Can you work these out from the model? Positions are in its coordinate system, mm. A direction names the side the tool comes from. Coordinates: 2 decimals unless noted, no trailing zeros. Loops run counter-clockwise (first coordinate to the right, second up) from the corner with the lowest first, then second, coordinate; pieces in that order, holes last. Notation, with made-up numbers: M 28.25,43 L 33.25,43 A29 ccw 33.25,73 Z; hole C -19,43 d8. An arc over 180 degrees is marked long. Return JSON: item names as keys, results as strings. Group by question number.
```python
from build123d import *

# Parameters (mm, degrees)
SKETCH1_W           = 119
SKETCH1_H           = 40
BOSS_EXTRUDE1_DEPTH = 4
SKETCH2_W           = 125
SKETCH2_H           = 46
SKETCH2_W_2         = 119
SKETCH2_H_2         = 40
BOSS_EXTRUDE2_DEPTH = 44
SKETCH3_W           = 58.2
SKETCH3_H           = 40
BOSS_EXTRUDE3_DEPTH = 3
SKETCH4_W           = 28
SKETCH4_H           = 40
BOSS_EXTRUDE4_DEPTH = 1.5
SKETCH5_R           = 4
BOSS_EXTRUDE5_DEPTH = 12
SKETCH6_R           = 11.5
SKETCH6_R_2         = 4
CUT_EXTRUDE1_DEPTH  = 3
SKETCH7_R           = 11.5
SKETCH7_R_2         = 9
CUT_EXTRUDE2_DEPTH  = 1


with BuildPart() as part:
    # Sketch1 → Boss-Extrude1 (new body)
    with BuildSketch(Plane(origin=(0, 0, 0), x_dir=(1, 0, 0), z_dir=(0, 1, 0))):
        Rectangle(SKETCH1_W, SKETCH1_H)
    extrude(amount=BOSS_EXTRUDE1_DEPTH)

    # Sketch2 → Boss-Extrude2 (add)
    with BuildSketch(Plane(origin=(0, 0, 0), x_dir=(1, 0, 0), z_dir=(0, 1, 0))):
        Rectangle(SKETCH2_W, SKETCH2_H)
        Rectangle(SKETCH2_W_2, SKETCH2_H_2, mode=Mode.SUBTRACT)
    extrude(amount=BOSS_EXTRUDE2_DEPTH)

    # Sketch3 → Boss-Extrude3 (add)
    with BuildSketch(Plane(origin=(0, 4, 0), x_dir=(1, 0, 0), z_dir=(0, 1, 0))):
        with Locations((30.4, 0)):
            Rectangle(SKETCH3_W, SKETCH3_H)
    extrude(amount=BOSS_EXTRUDE3_DEPTH)

    # Sketch4 → Boss-Extrude4 (add)
    with BuildSketch(Plane(origin=(0, 7, 0), x_dir=(1, 0, 0), z_dir=(0, 1, 0))):
        with Locations((15.3, 0)):
            Rectangle(SKETCH4_W, SKETCH4_H)
    extrude(amount=BOSS_EXTRUDE4_DEPTH)

    # Sketch5 → Boss-Extrude5 (add)
    with BuildSketch(Plane.XZ):
        with Locations((39.5, 0)):
            Circle(SKETCH5_R)
    extrude(amount=BOSS_EXTRUDE5_DEPTH)

    # Sketch6 → Cut-Extrude1 (cut)
    with BuildSketch(Plane.XZ):
        with Locations((39.5, 0)):
            Circle(SKETCH6_R)
        with Locations((39.5, 0)):
            Circle(SKETCH6_R_2, mode=Mode.SUBTRACT)
    extrude(amount=-CUT_EXTRUDE1_DEPTH, mode=Mode.SUBTRACT)

    # Sketch7 → Cut-Extrude2 (cut)
    with BuildSketch(Plane.XZ.offset(-3)):
        with Locations((39.5, 0)):
            Circle(SKETCH7_R)
        with Locations((39.5, 0)):
            Circle(SKETCH7_R_2, mode=Mode.SUBTRACT)
    extrude(amount=-CUT_EXTRUDE2_DEPTH, mode=Mode.SUBTRACT)


solid = part.part
```
1) Suppose I cut it at C-C, the plane z = 0. List the corners of the cut face in (x, y) for me, then the cut area to 3 significant figures.
2) If I drill on line 1 (Z direction, x = 39.5, y = 0.85); line 2 (Z direction, x = -6.5, y = 15.5); line 3 (X direction, y = 17, z = 16.5), over which ranges is the centre line in solid material (lowest first)? Write a range as from..to.
3) Suppose I cut it at D-D, the plane z = 13. List the corners of the cut face in (x, y) for me, then the cut area to 3 significant figures.
4) If we mould it in two halves opening along Z, with no side actions, what happens to faces 4 (the face through (-1, 22, -23)), 5 (the face through (39, -12, 0)), 6 (the face through (59.5, 25, 0))? For each: +Z half, -Z half, draft (parallel to the pull), parting line (faces both ways), or undercut.
5) Suppose I cut it at A-A, the plane y = 12.5. List the corners of the cut face in (x, z) for me, then the cut area to 3 significant figures.
6) For pin 1 (14 mm diameter, centred on x = 8.5, z = 9, fed in from +Y); pin 2 (12 mm diameter, centred on x = 39, z = 1, fed in from +Y); pin 3 (18.5 mm diameter, centred on x = 38, z = 5.5, fed in from -Y), each with a flat end and sliding along its axis, tell me the tip position at first contact or that it passes through.
7) Suppose I cut it at B-B, the plane x = 39.5. List the corners of the cut face in (y, z) for me, then the cut area to 3 significant figures.
8) For faces 1 (the face through (62.5, 22, 0)), 2 (the face through (-30, 4, 0)), 3 (the face through (43.4, 3, -1.9)), which set-ups out of +Z, -Z, +X, -X, +Y, -Y let a thin tool reach every point of the face, with its end or its side?
Returned:
{
 "1": {"outline": "M -62.5,0 L 28,0 L 28,4 L 30.5,4 L 30.5,3 L 35.5,3 L 35.5,-12 L 43.5,-12 L 43.5,3 L 48.5,3 L 48.5,4 L 51,4 L 51,0 L 62.5,0 L 62.5,44 L 59.5,44 L 59.5,7 L 29.3,7 L 29.3,8.5 L 1.3,8.5 L 1.3,4 L -59.5,4 L -59.5,44 L -62.5,44 Z", "area": "1,000 mm²"},
 "2": {"line 1": "z = -23..-11.5, -4..4, 11.5..23", "line 2": "z = -23..-20, 20..23", "line 3": "x = -62.5..-59.5, 59.5..62.5"},
 "3": {"outline": "M -62.5,0 L 62.5,0 L 62.5,44 L 59.5,44 L 59.5,7 L 29.3,7 L 29.3,8.5 L 1.3,8.5 L 1.3,4 L -59.5,4 L -59.5,44 L -62.5,44 Z", "area": "957 mm²"},
 "4": {"face 4": "-Z half", "face 5": "draft", "face 6": "undercut"},
 "5": {"outline": "M -62.5,-23 L 62.5,-23 L 62.5,23 L -62.5,23 Z; hole M -59.5,-20 L 59.5,-20 L 59.5,20 L -59.5,20 Z", "area": "990 mm²"},
 "6": {"pin 1": "stops at y = 8.5", "pin 2": "stops at y = 7", "pin 3": "stops at y = -12"},
 "7": {"outline": "M -12,-4 L 3,-4 L 3,-9 L 4,-9 L 4,-11.5 L 0,-11.5 L 0,-23 L 44,-23 L 44,-20 L 7,-20 L 7,20 L 44,20 L 44,23 L 0,23 L 0,11.5 L 4,11.5 L 4,9 L 3,9 L 3,4 L -12,4 Z", "area": "590 mm²"},
 "8": {"face 1": "+Z, -Z, +X, +Y, -Y", "face 2": "+Y", "face 3": "-Y"}
}
